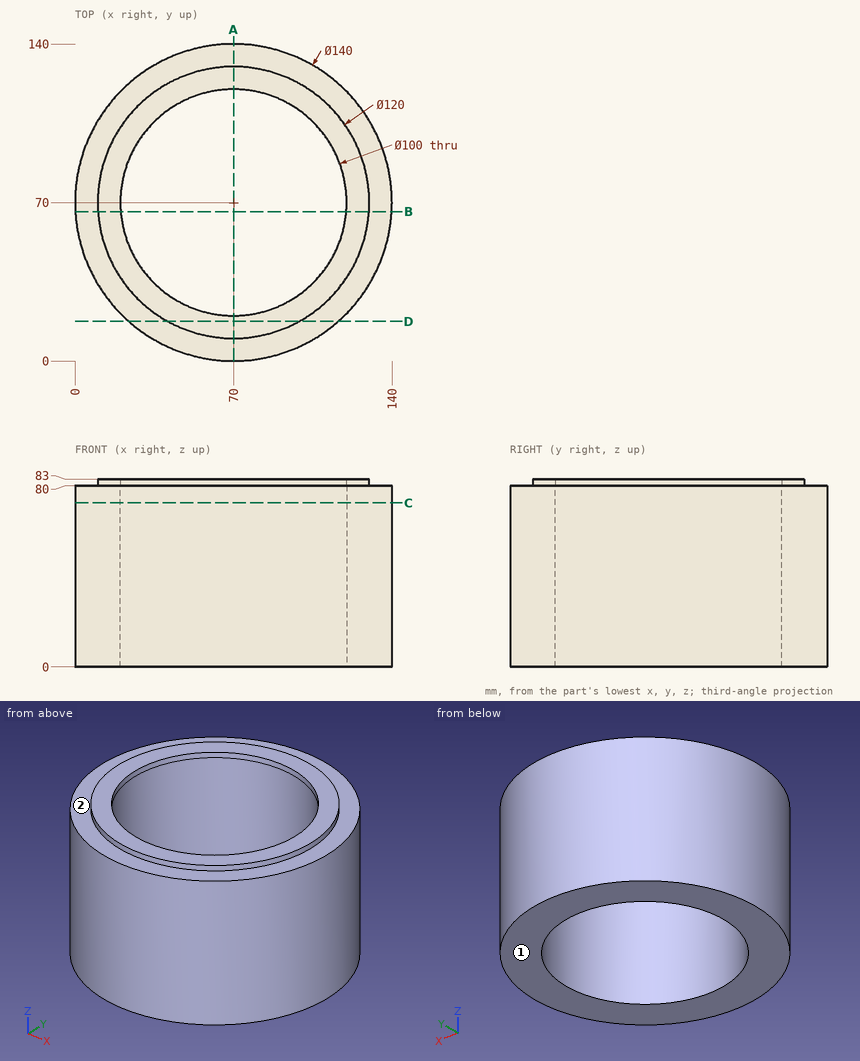
Answer from the drawing. Dimensions are ordinates in mm from the lowest x, y and z of the part. A direction names the side the tool comes from. Round coordinates to 2 decimals unless told otherwise and drop trailing zeros. Write each loop counter-clockwise with the first axis right and the second up, starting at its lowest first coordinate (ties: lowest second). Pieces come first, ordered by that corner, then holes. Notation, with made-up numbers: M 18,-26.75 L 26,-26.75 A18 cw 26,7.25 Z; hole C 39.5,19 d10. An arc over 180 degrees is marked long. Write each question's results on one line, items separated by ' | '. Start each with the question number.
Item 1: Straight lines are drawn through the part: probe 1 along Y at (x, z) = (70, 81); probe 2 along Y at (x, z) = (70, 33); probe 3 along Z at (x, y) = (10, 37). For each, find the intervals that lie inside material, in ascending order.
Item 2: Find section A-A on x = 70. Write down the section's boundary in (y, z), and give its area (3 significant figures).
Item 3: Which of the six approach directions +Z, -Z, +X, -X, +Y, -Y give full straight-line access (tool end or side, diameter ignored) to the marked faces 1 and 2?
Item 4: Find section C-C on z = 72.5. Write down the section's boundary in (x, y), and give its area (3 significant figures).
Item 5: Given pin 1 Ø10 at (x, z) = (94, 38) entering from -Y; pin 2 Ø1 at (x, z) = (96.5, 56) entering from +Y; pin 3 Ø1.5 at (x, z) = (31.5, 73) entering from -Y, each flat-ended and moving along its own axis, determine where each tip first touches the part or whether it passes through.
Item 6: Find section B-B on y = 66. Write down the section's boundary in (x, z), and give its area (3 significant figures).
Item 7: Find section D-D on y = 17.5. Write down the section's boundary in (x, z), and give its area (3 significant figures).
Answer block:
1) probe 1: y = 10 to 20, 120 to 130 | probe 2: y = 0 to 20, 120 to 140 | probe 3: z = 0 to 80
2) outline: M 0,0 L 20,0 L 20,83 L 10,83 L 10,80 L 0,80 Z; M 120,0 L 140,0 L 140,80 L 130,80 L 130,83 L 120,83 Z | area: 3,260 mm²
3) face 1: -Z, +X, -X, +Y, -Y | face 2: +Z
4) outline: C 70,70 d140; hole C 70,70 d100 | area: 7,540 mm²
5) pin 1: stops at y = 2.63 | pin 2: stops at y = 134.99 | pin 3: stops at y = 11.05
6) outline: M 0.11,0 L 20.16,0 L 20.16,83 L 10.13,83 L 10.13,80 L 0.11,80 Z; M 119.84,0 L 139.89,0 L 139.89,80 L 129.87,80 L 129.87,83 L 119.84,83 Z | area: 3,270 mm²
7) outline: M 23.7,0 L 116.3,0 L 116.3,80 L 99.05,80 L 99.05,83 L 40.95,83 L 40.95,80 L 23.7,80 Z | area: 7,580 mm²
